CAD build for the part. Positions are in the model's coordinates, mm. Coordinates: 2 decimals unless noted, no trailing zeros. Loops run counter-clockwise (first coordinate to the right, second up) from the corner with the lowest first, then second, coordinate; pieces in that order, holes last. Notation, with made-up numbers: (88.25, 73) -> (111.25, 73) arc R21 cw to (111.25, 108) -> close; hole circle Ø11 at (87, -15.75). An arc over 180 degrees is marked (long way). Write item = value, one per line. Start each with the question number.
(1) Drill centre lines: line 1 (Z direction, x = 0, y = 1.5); line 2 (Z direction, x = -81.5, y = 0.85); line 3 (Z direction, x = 18, y = 3.7). Where is each one in solid material? Low to high. Write a range as from..to.
(2) Band-saw the part on C-C (y = 3.1). Write the cut outline in (x, z).
(3) Flat gauge pins, fed straight in: P1, Ø6, axis at x = -29.5, z = 49.5, coming from the -Y side; P2, Ø1, axis at x = -55, y = 2.5, coming from the +Z side. Where does each tip first touch, or does it go through?
(4) Band-saw the part on D-D (z = 26). Write the cut outline in (x, y), and give its area (3 significant figures).
(5) Band-saw the part on B-B (x = 0). Write the cut outline in (y, z), and give its area (3 significant figures).
(6) Band-saw the part on A-A (z = 0). Write the cut outline in (x, y).
(7) Pull direction X, two halves, no side cores. Call faces 1 (the face through (-99.59, 2.03, 14.8)), 2 (the face through (42.15, 2.03, -41.99)), 3 (the face through (1.107, 1.972, 76.572)): +X half, -X half, draft (parallel to the pull), parting line (faces both ways), or undercut.
Autodesk Inventor part; units mm, degrees
ref_plane "YZ Plane" through (0, 0, 0) normal (1, 0, 0) x (0, 1, 0)
ref_plane "XZ Plane" through (0, 0, 0) normal (0, 1, 0) x (-1, 0, 0)
ref_plane "XY Plane" through (0, 0, 0) normal (0, 0, 1) x (1, 0, 0)
sketch "Sketch1" plane through (0, 0, 0) normal (0, 1, 0) x (-1, 0, 0)
  line L0 (40, 40) -> (-40, 40) construction
  line L1 (-40, 40) -> (-40, -40) construction
  line L2 (-40, -40) -> (40, -40) construction
  line L3 (40, -40) -> (40, 40) construction
  line L4 (-40, 40) -> (40, -40) construction
  line L5 (100, -45) -> (-100, -45)
  line L6 (-100, -45) -> (-100, 100)
  line L7 (-100, 100) -> (100, 100)
  line L8 (100, 100) -> (100, -45)
  circle A0 centre (85, 0) radius 8.5
  circle A1 centre (0, 85) radius 8.5
  circle A2 centre (-85, 0) radius 8.5
  line L9 (0, 40) -> (0, -40) construction
  line L10 (100, 15) -> (20, 100)
  line L11 (-20, 100) -> (-100, 15)
  line L12 (100, -15) -> (71.7647, -45)
  line L13 (-100, -15) -> (-71.7647, -45)
  line L14 (0, 0) -> (-40, 0) construction
  line L15 (-45, -45) -> (-45, 73.4375)
  point P0 (0, 0)
  point P1 (0, 0)
  dimension "d2" = 80
  dimension "d3" = 80
  dimension "d17" = 5
  dimension "d18" = 17
  dimension "d19" = 45
  dimension "d20" = 45
  dimension "d21" = 40
  dimension "d22" = 15
  dimension "d23" = 15
  dimension "d24" = 30
  dimension "d26" = 5
extrude "Plate1" add sketch "Sketch1" along normal blind 4 contours L5 L15 L11 L7 L10 L8 L12
fillet "Corner Round2" radius 6 6 edges at (-20, 2, 100) (20, 2, 100) (-100, 2, 15) (-100, 2, -15) (-71.7647, 2, -45) (45, 2, 73.4375)
fillet "Corner Round4" radius 10 1 edges at (45, 2, -45)
equation "\"d20\" = d19"
equation "\"d23\" = d22"
equation "\"d26\" = d17"
equation "\"d6\" = Thickness"
equation "\"BendReliefWidth\" = Thickness"
equation "\"BendReliefDepth\" = 0.5 * Thickness"
equation "\"CornerReliefSize\" = 4 * Thickness"
equation "\"MinimumRemnant\" = 2 * Thickness"
equation "\"TransitionRadius\" = BendRadius"
equation "\"JacobiRadiusSize\" = BendRadius"
equation "\"GapSize\" = Thickness"
properties part number "MSC 902 FLANGE FRAME HEEL" material "Stainless Steel"
Findings below:
q1.line_1 = -45..76.5, 93.5..100
q1.line_2 = -34.66..-7.75, 7.75..34.66
q1.line_3 = -45..99.97
q2.outline = (-100, -12.62) arc R6 ccw to (-98.37, -16.73) -> (-73.54, -43.11) arc R6 ccw to (-69.17, -45) -> (35, -45) arc R10 ccw to (45, -35) -> (45, 71.06) arc R6 ccw to (43.37, 75.17) -> (21.78, 98.11) arc R6 ccw to (17.41, 100) -> (-17.41, 100) arc R6 ccw to (-21.78, 98.11) -> (-98.37, 16.73) arc R6 ccw to (-100, 12.62) -> close; hole circle Ø17 at (-85, 0); hole circle Ø17 at (0, 85)
q3.P1 = 0
q3.P2 = 63.34
q4.outline = (-89.65, 0) -> (45, 0) -> (45, 4) -> (-89.65, 4) -> close
q4.area = 539 mm²
q5.outline = (0, -45) -> (4, -45) -> (4, 76.5) -> (0, 76.5) -> close; (0, 93.5) -> (4, 93.5) -> (4, 100) -> (0, 100) -> close
q5.area = 512 mm²
q6.outline = (-100, 0) -> (-93.5, 0) -> (-93.5, 4) -> (-100, 4) -> close; (-76.5, 0) -> (45, 0) -> (45, 4) -> (-76.5, 4) -> close
q7.face_1 = -X half
q7.face_2 = +X half
q7.face_3 = undercut
